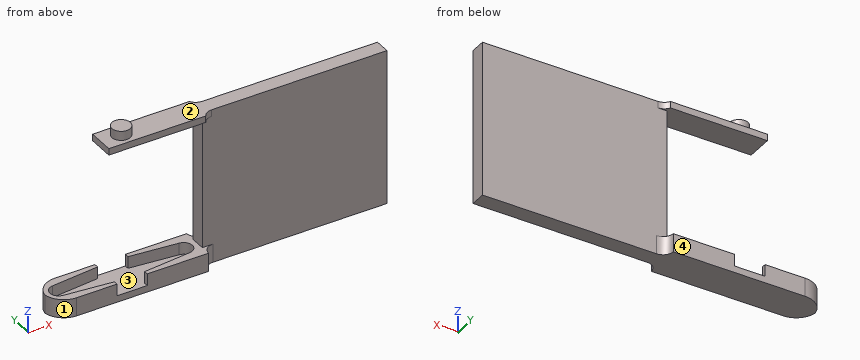
```python
from build123d import *

# Parameters (mm, degrees)
SKETCH1_W            = 29
SKETCH1_H            = 6.75
BOSS_EXTRUDE10_DEPTH = 3.5
SKETCH1_16_R         = 0.291434634
BOSS_EXTRUDE15_DEPTH = 1.25
SKETCH1_17_W         = 35
SKETCH1_17_H         = 2.924143722
BOSS_EXTRUDE17_DEPTH = 29.5
BOSS_EXTRUDE18_DEPTH = 1.25
SKETCH2_9_R          = 1.75
BOSS_EXTRUDE19_DEPTH = 1.75
FILLET1_R            = 2
FILLET2_R            = 4
SKETCH3_W            = 5.75
SKETCH3_H            = 0.795101344
CUT_EXTRUDE1_DEPTH   = 2.25


with BuildPart() as part:
    # Sketch1 → Boss-Extrude10 (new body)
    with BuildSketch(Plane.XY):
        with Locations((0, 3.375)):
            Rectangle(SKETCH1_W, SKETCH1_H)
        with BuildLine():
            Line((-12.018477316, 5.016376067), (0, 6.25))
            Line((0, 6.25), (12.018477316, 5.016376067))
            ThreePointArc((12.018477316, 5.016376067), (13.5, 3.375), (12.018477316, 1.733623933))
            Line((12.018477316, 1.733623933), (0, 0.5))
            Line((0, 0.5), (-12.018477316, 1.733623933))
            ThreePointArc((-12.018477316, 1.733623933), (-13.5, 3.375), (-12.018477316, 5.016376067))
        make_face(mode=Mode.SUBTRACT)
    extrude(amount=BOSS_EXTRUDE10_DEPTH)

    # Sketch1<16> → Boss-Extrude15 (add)
    # profile 1 of 9: a face of its own
    with BuildSketch(Plane.XY):
        with BuildLine():
            Line((-0.584049273, 6.190050878), (-12.018477316, 5.016376067))
            ThreePointArc((-12.018477316, 5.016376067), (-13.5, 3.375), (-12.018477316, 1.733623933))
            Line((-12.018477316, 1.733623933), (-0.584049273, 0.559949122))
            ThreePointArc((-0.584049273, 0.559949122), (-2.875, 3.375), (-0.584049273, 6.190050878))
        make_face()
        with Locations((-11.85, 3.375)):
            Circle(SKETCH1_16_R, mode=Mode.SUBTRACT)
        with Locations((-9.813185408, 3.375)):
            Circle(SKETCH1_16_R, mode=Mode.SUBTRACT)
        with Locations((-7.776370816, 3.375)):
            Circle(SKETCH1_16_R, mode=Mode.SUBTRACT)
    # profile 2 of 9: a face of its own
    with BuildSketch(Plane.XY):
        with Locations((-11.85, 3.375)):
            Circle(SKETCH1_16_R)
    # profile 3 of 9: a face of its own
    with BuildSketch(Plane.XY):
        with Locations((-7.776370816, 3.375)):
            Circle(SKETCH1_16_R)
    # profile 4 of 9: a face of its own
    with BuildSketch(Plane.XY):
        with Locations((-9.813185408, 3.375)):
            Circle(SKETCH1_16_R)
    # profile 5 of 9: a face of its own
    with BuildSketch(Plane.XY):
        with BuildLine():
            Line((0, 6.25), (-0.584049273, 6.190050878))
            ThreePointArc((-0.584049273, 6.190050878), (-2.875, 3.375), (-0.584049273, 0.559949122))
            Line((-0.584049273, 0.559949122), (0, 0.5))
            Line((0, 0.5), (0.584049273, 0.559949122))
            ThreePointArc((0.584049273, 0.559949122), (2.229884152, 1.56027091), (2.875, 3.375))
            ThreePointArc((2.875, 3.375), (2.229884152, 5.18972909), (0.584049273, 6.190050878))
            Line((0.584049273, 6.190050878), (0, 6.25))
        make_face()
    # profile 6 of 9: a face of its own
    with BuildSketch(Plane.XY):
        with BuildLine():
            Line((12.018477316, 5.016376067), (0.584049273, 6.190050878))
            ThreePointArc((0.584049273, 6.190050878), (2.229884152, 5.18972909), (2.875, 3.375))
            ThreePointArc((2.875, 3.375), (2.229884152, 1.56027091), (0.584049273, 0.559949122))
            Line((0.584049273, 0.559949122), (12.018477316, 1.733623933))
            ThreePointArc((12.018477316, 1.733623933), (13.5, 3.375), (12.018477316, 5.016376067))
        make_face()
        with Locations((7.776370816, 3.375)):
            Circle(SKETCH1_16_R, mode=Mode.SUBTRACT)
        with Locations((9.813185408, 3.375)):
            Circle(SKETCH1_16_R, mode=Mode.SUBTRACT)
        with Locations((11.85, 3.375)):
            Circle(SKETCH1_16_R, mode=Mode.SUBTRACT)
    # profile 7 of 9: a face of its own
    with BuildSketch(Plane.XY):
        with Locations((11.85, 3.375)):
            Circle(SKETCH1_16_R)
    # profile 8 of 9: a face of its own
    with BuildSketch(Plane.XY):
        with Locations((9.813185408, 3.375)):
            Circle(SKETCH1_16_R)
    # profile 9 of 9: a face of its own
    with BuildSketch(Plane.XY):
        with Locations((7.776370816, 3.375)):
            Circle(SKETCH1_16_R)
    extrude(amount=BOSS_EXTRUDE15_DEPTH)

    # Sketch1<17> → Boss-Extrude17 (add)
    with BuildSketch(Plane.XY):
        with Locations((32, 3.375)):
            Rectangle(SKETCH1_17_W, SKETCH1_17_H)
    extrude(amount=BOSS_EXTRUDE17_DEPTH)

    # Sketch2 → Boss-Extrude18 (add)
    with BuildSketch(Plane.XY.offset(29.5)):
        Polygon((13.5, 5.875), (-3.875, 5.875), (-3.875, 0.875), (14.5, 0.875), (14.5, 5.875), align=None)
    extrude(amount=-BOSS_EXTRUDE18_DEPTH)

    # Sketch2<9> → Boss-Extrude19 (add)
    with BuildSketch(Plane.XY.offset(29.5)):
        with Locations((0, 3.375)):
            Circle(SKETCH2_9_R)
    extrude(amount=BOSS_EXTRUDE19_DEPTH)

    # Fillet1
    # the kernel refuses this fillet: 2 mm, written as the material it adds along each edge
    with BuildSketch(Plane(origin=(14.5, 1.912928139, 0), x_dir=(0, -1, 0), z_dir=(0, 0, 1))) as fillet1_piece_1:
        with BuildLine():
            CenterArc((2, 1.998103724), FILLET1_R, 180, 87.504786267)
            Line((0, 1.998103724), (0, 0))
            Line((0, 0), (1.912928139, 0))
        make_face()
    extrude(amount=3.5)
    with BuildSketch(Plane(origin=(14.5, 4.837071861, 0), x_dir=(1, 0, 0), z_dir=(0, 0, 1))) as fillet1_piece_2:
        with BuildLine():
            CenterArc((1.998103724, 2), FILLET1_R, 182.495213733, 87.504786267)
            Line((0, 1.912928139), (0, 0))
            Line((0, 0), (1.998103724, 0))
        make_face()
    extrude(amount=3.5)
    with BuildSketch(Plane(origin=(14.5, 1.912928139, 28.25), x_dir=(1, 0, 0), z_dir=(0, 0, 1))) as fillet1_piece_3:
        with BuildLine():
            CenterArc((1.753401761, -2), FILLET1_R, 90, 61.246917848)
            Line((0, -1.037928139), (0, 0))
            Line((0, 0), (1.753401761, 0))
        make_face()
    extrude(amount=1.25)
    with BuildSketch(Plane(origin=(14.5, 4.837071861, 28.25), x_dir=(1, 0, 0), z_dir=(0, 0, 1))) as fillet1_piece_4:
        with BuildLine():
            CenterArc((1.753401761, 2), FILLET1_R, 208.753082152, 61.246917848)
            Line((0, 1.037928139), (0, 0))
            Line((0, 0), (1.753401761, 0))
        make_face()
    extrude(amount=1.25)

    # Fillet2
    # the kernel refuses this fillet: 4 mm, written as the material it takes off along each edge
    with BuildSketch(Plane(origin=(-14.5, 6.75, -10), x_dir=(0, -1, 0), z_dir=(0, 0, 1)), Plane(origin=(-14.5, 0, -10), x_dir=(1, 0, 0), z_dir=(0, 0, 1))) as fillet2_piece_1:
        with BuildLine():
            CenterArc((FILLET2_R, FILLET2_R), FILLET2_R, 180, 90)
            Line((0, FILLET2_R), (0, 0))
            Line((0, 0), (FILLET2_R, 0))
        make_face()
    extrude(amount=23.5, mode=Mode.SUBTRACT)

    # Sketch3 → Cut-Extrude1 (cut)
    with BuildSketch(Plane.XY.offset(3.5)):
        with Locations((0, 0.397550672)):
            Rectangle(SKETCH3_W, SKETCH3_H)
        with Locations((0, 6.352449328)):
            Rectangle(SKETCH3_W, SKETCH3_H)
    extrude(amount=-CUT_EXTRUDE1_DEPTH, mode=Mode.SUBTRACT)


solid = part.part
```
The model under review builds one solid part; all positions refer to its coordinate system, in mm. Face numbers are marked on the shaded views. Round coordinates to 2 decimals unless told otherwise and drop trailing zeros. Loops run counter-clockwise (first coordinate to the right, second up) from the corner with the lowest first, then second, coordinate; pieces in that order, holes last.
Item 1: For line 1 (Z direction, x = 3.5, y = 1.25); line 2 (Z direction, x = -1, y = 2.25); line 3 (Z direction, x = -10, y = 3.5), list the stretches that pass through material, from the lowest coordinate up.
Determined:
line 1: z = 0 to 1.25, 28.25 to 29.5
line 2: z = 0 to 1.25, 28.25 to 31.25
line 3: z = 0 to 1.25
Item 2: Clearance check with flat-ended pins moving along their axes: pin 1 Ø0.9 at (y, z) = (0.5, 2) entering from +X; pin 2 Ø1 at (y, z) = (4.5, 20.5) entering from -X; pin 3 Ø0.9 at (y, z) = (6.5, 2) entering from +X. State where each tip first meets the part, or that it passes through.
Determined:
pin 1: stops at x = 14.79
pin 2: stops at x = 14.5
pin 3: stops at x = 14.66
Item 3: Take a section at A-A (x = 10.5). Write out the cut boundary in (y, z) (3 decimals), then the cut area to 3 significant figures.
Determined:
outline: (0, 0) - (6.75, 0) - (6.75, 3.5) - (5.172, 3.5) - (5.172, 1.25) - (1.578, 1.25) - (1.578, 3.5) - (0, 3.5) - close; (0.875, 28.25) - (5.875, 28.25) - (5.875, 29.5) - (0.875, 29.5) - close
area: 21.8 mm2
Item 4: Mouldability with a two-part tool opening along Y and no side actions: class the marked faces 1, 2, 3 and 4 as released by +Y, released by -Y, zero draft, split by the parting line, or undercut.
Determined:
face 1: released by -Y
face 2: zero draft
face 3: undercut
face 4: released by +Y
Item 5: Take a section at D-D (x = 44.5). Write out the cut boundary in (y, z).
Determined:
outline: (1.91, 0) - (4.84, 0) - (4.84, 29.5) - (1.91, 29.5) - close
Item 6: Take a section at C-C (x = 0). Write out the cut boundary in (y, z) (3 decimals).
Determined:
outline: (0, 0) - (6.75, 0) - (6.75, 1.25) - (0, 1.25) - close; (0.875, 28.25) - (5.875, 28.25) - (5.875, 29.5) - (5.125, 29.5) - (5.125, 31.25) - (1.625, 31.25) - (1.625, 29.5) - (0.875, 29.5) - close
Item 7: Take a section at B-B (z = 6). Write out the cut boundary in (x, y), then the cut area to 3 significant figures.
Determined:
outline: (14.5, 1.91) - (49.5, 1.91) - (49.5, 4.84) - (14.5, 4.84) - close
area: 102 mm2
